Design review of the part built by this model. Coordinates are the model's own, in mm. A direction names the side the tool comes from. Coordinates: 2 decimals unless noted, no trailing zeros. Loops run counter-clockwise (first coordinate to the right, second up) from the corner with the lowest first, then second, coordinate; pieces in that order, holes last. Notation, with made-up numbers: (49.25, 3.25) -> (88.25, 3.25) arc R29 ccw to (88.25, 41.25) -> close; hole circle Ø11 at (16.5, 2.5). An arc over 180 degrees is marked (long way). Use CSV: the item, a comma, the result in double quotes.
```python
from build123d import *

# Parameters (mm, degrees)
F3_T = -1
F4_T = 0.2


# Not quite as in the source:
# - a shell that OpenCascade refuses in one call is made with other operations: the cavity is built on its own and cut out


with BuildPart() as f2:
    # F0 (on Right) → F2 (revolve)
    with BuildSketch(Plane.YZ):
        with BuildLine():
            Line((15, 37.0809924355), (0, 37.0809924355))
            Line((0, 37.0809924355), (0, 0))
            Line((0, 0), (0, -3.1108935364))
            Line((0, -3.1108935364), (42.2, -3.1108935364))
            Line((42.2, -3.1108935364), (42.2, 0))
            Line((42.2, 0), (40, 0))
            ThreePointArc((40, 0), (33.1662479036, 22.360679775), (15, 37.0809924355))
        make_face()
    revolve(axis=Axis((0, 0, 9.5782782882), (0, 0, -1)))

    # F3
    f3_openings = [f2.faces().sort_by_distance(p)[0] for p in [
        (0, 0, 37.080992),
        (0, 0, -3.110894),
    ]]
    offset(amount=F3_T, openings=f3_openings, kind=Kind.INTERSECTION)

    # F4: shell of thickness 0.2, made by hand


with BuildPart() as f4_core1:
    # F4_t2: copy of F2
    add(f2.part)

    # the walls: a layer under each face that stays
    f4_faces = [f4_core1.faces().sort_by_distance(p)[0] for p in [
        (0, -42.2, -1.5554467682),
        (-11.2533333333, -39.3866666667, 0),
        (0, -33.1662479036, 22.360679775),
        (-10, -10, 37.0809924355),
        (0, -31.8525104905, 22.5037235909),
        (-20.3185185185, -36.925, -3.1108935364),
        (-10.9866666667, -38.4533333333, -1),
    ]]
    thicken(f4_faces, amount=-F4_T, mode=Mode.SUBTRACT)

    # F4_s3 → F4_t4 (revolve, cut)
    with BuildSketch(Plane.YZ):
        Polygon((40.002, 0.002), (40, -0.2), (39.8, -0.2), (39.8, 0), align=None)
    revolve(axis=Axis((0, 0, 0), (0, 0, -1)), mode=Mode.SUBTRACT)


with BuildPart() as f2_1:
    add(f2.part)

    # what is left inside the walls is the cavity
    f4_cavity = [f4_core1.part.solids().sort_by_distance(p)[0] for p in [
        (0, -36.186898, 15.076644),
    ]]
    add(f4_cavity, mode=Mode.SUBTRACT)


solid = f2_1.part
```
Item 1: Add section D-D (z = 31). Give the boundary of the cut face in (x, y) (1 decimal).
Checked values:
outline,"circle Ø50.6 at (0, 0); circle Ø48 at (0, 0); hole circle Ø49.9 at (0, 0); hole circle Ø47.3 at (0, 0)"
Item 2: Add section A-A (x = -35). Give the boundary of the cut face in (y, z).
Checked values:
outline,"(-23.58, -3.11) -> (-21.74, -3.11) -> (-21.74, -2.91) -> (-23.22, -2.91) -> (-23.22, -0.2) -> (-18.95, -0.2) -> (-18.95, 0) arc R18.95 cw to (18.95, 0) -> (18.95, -0.2) -> (23.22, -0.2) -> (23.22, -2.91) -> (21.74, -2.91) -> (21.74, -3.11) -> (23.58, -3.11) -> (23.58, 0) -> (19.36, 0) arc R19.36 ccw to (-19.36, 0) -> (-23.58, 0) -> close; (-21.74, -1) -> (-17.18, -1) arc R17.2 cw (long way) to (17.18, -1) -> (21.74, -1) -> (21.74, -0.8) -> (17.64, -0.8) arc R17.65 ccw (long way) to (-17.64, -0.8) -> (-21.74, -0.8) -> close"
Item 3: Machinability: for faces 5 (the face through (-36.4, 15.1, -0.8)), 6 (the face through (-40.4, -9.2, -3.111)), which of the approach directions +Z, -Z, +X, -X, +Y, -Y give a long, thin tool a straight path to every point of the face, cutting with its end or side? Answer none if there is none.
Checked values:
face 5,"none"
face 6,"-Z, +X, -X, +Y, -Y"
Item 4: To check wall thickness, follow line 1 along X through (y, z) = (0, -0.1); line 2 along Z through (x, y) = (36, 18); line 3 along Y through (x, z) = (-1, 13). State the ranges of each line that lie inside material, in increasing order.
Checked values:
line 1,"-42.2 to -39.8, -39.2 to -39, 39 to 39.2, 39.8 to 42.2"
line 2,"-1 to -0.8, -0.2 to 0"
line 3,"-37.82 to -37.6, -36.97 to -36.76, 36.76 to 36.97, 37.6 to 37.82"
Item 5: Clearance check with flat-ended pins moving along their axes: pin 1 (6 mm diameter, centred on x = -1.5, z = 19, fed in from +Y); pin 2 (6 mm diameter, centred on y = -20.5, z = 19.5, fed in from -X); pin 3 (2 mm diameter, centred on x = -6, y = -24, fed in from -Z). State where each tip first meets the part, or that it passes through.
Checked values:
pin 1,"y = 36.63"
pin 2,"x = -30.99"
pin 3,"z = 29.3"
Item 6: Draft analysis for pull direction Z (two halves, no side actions). For faces 1 (the face through (12.68, 40.25, -1.53)), 2 (the face through (-31, -28, -2.911)), 3 (the face through (-36.4, 15.1, -1)), 4 (the face through (-37.3, 15.4, 0)), state which applies: pulls with the +Z half, pulls with the -Z half, needs draft (parallel to the pull), parting line crosses it, or undercut.
Checked values:
face 1,"needs draft"
face 2,"undercut"
face 3,"pulls with the -Z half"
face 4,"pulls with the +Z half"
